Build history of the part. All positions in model axes, mm. Coordinates: 2 decimals unless noted, no trailing zeros. Loops run counter-clockwise (first coordinate to the right, second up) from the corner with the lowest first, then second, coordinate; pieces in that order, holes last.
(1) Wall check: L1, parallel to Y at x = 6.5, z = 15; L2, parallel to Z at x = 9.25, y = -218.79; L3, parallel to Y at x = 25, z = 18.25. Give the ranges that are in metal, low to high.
(2) Slice it at B-B (y = -218.79). Give the cut face in (x, z).
(3) Slice it at A-A (z = 15). Give the cut face in (x, y).
(4) Two-plate mould, pull along Y, no slides. Class faces 1 (the face through (15.21, -214.885, 14.133)), 2 (the face through (30, -118, 15)), 3 (the face through (15, -240, 15)): pulls with the +Y half, pulls with the -Y half, needs draft (parallel to the pull), parting line crosses it, or undercut.
from build123d import *

# Parameters (mm, degrees)
SKETCH_W     = 30
SKETCH_H     = 30
PAD_DEPTH    = 240
SKETCH001_R  = 4
POCKET_DEPTH = 30.001


with BuildPart() as part:
    # Sketch → Pad (new body)
    with BuildSketch(Plane.XZ):
        with Locations((15, 15)):
            Rectangle(SKETCH_W, SKETCH_H)
    extrude(amount=PAD_DEPTH)

    # Sketch001 (on Face2 of Pad) → Pocket (cut, through all)
    with BuildSketch(Plane(origin=(30, 0, 0), x_dir=(0, 0, 1), z_dir=(1, 0, 0))):
        with Locations((15, 218.79)):
            Circle(SKETCH001_R)
    extrude(amount=-POCKET_DEPTH, mode=Mode.SUBTRACT)


solid = part.part
Response values:
1. L1: y = -240 to -222.79, -214.79 to 0
1. L2: z = 0 to 11, 19 to 30
1. L3: y = -240 to -221.12, -216.46 to 0
2. outline: (0, 0) - (30, 0) - (30, 11) - (0, 11) - close; (0, 19) - (30, 19) - (30, 30) - (0, 30) - close
3. outline: (0, -240) - (30, -240) - (30, -222.79) - (0, -222.79) - close; (0, -214.79) - (30, -214.79) - (30, 0) - (0, 0) - close
4. face 1: undercut
4. face 2: needs draft
4. face 3: pulls with the -Y half
